Could you check a few things on this model? Use its own coordinates, in mm. A direction names the side the tool comes from. Give positions to 0.01 mm unless a question says otherwise; leave off trailing zeros. Order: outer loops, then holes, each group sorted by start corner. A loop starts at its lowest first (then second) coordinate and runs counter-clockwise, first axis right, second up. Notation, with made-up numbers: M 75,26 L 81,26 A11 cw 81,42 Z; hole C 48,36.5 d2. An arc over 180 degrees is marked long. Answer in a Markdown table with one row per item. Add a question column.
```python
from build123d import *

# Parameters (mm, degrees)
SKETCH_1_R      = 10
EXTRUDE_1_DEPTH = 2.5


with BuildPart() as part:
    # 草图1 → 凸台-拉伸1 (new body)
    with BuildSketch(Plane.XY):
        with BuildLine():
            Line((-24, -40), (-24, -50))
            ThreePointArc((-24, -50), (-15.443695821, -59.895238369), (-4.416851525, -52.857142857))
            ThreePointArc((-4.416851525, -52.857142857), (-2.974049354, -50.792865097), (-0.583592135, -50))
            Line((-0.583592135, -50), (0.583592135, -50))
            ThreePointArc((0.583592135, -50), (2.974049354, -50.792865097), (4.416851525, -52.857142857))
            ThreePointArc((4.416851525, -52.857142857), (15.443695821, -59.895238369), (24, -50))
            Line((24, -50), (24, -40))
            ThreePointArc((24, -40), (23.055385138, -35.757359313), (20.4, -32.316250915))
            ThreePointArc((20.4, -32.316250915), (16.416922293, -27.154588318), (15, -20.790627288))
            Line((15, -20.790627288), (15, 0))
            ThreePointArc((15, 0), (0, 15), (-15, 0))
            Line((-15, 0), (-15, -20.790627288))
            ThreePointArc((-15, -20.790627288), (-16.416922293, -27.154588318), (-20.4, -32.316250915))
            ThreePointArc((-20.4, -32.316250915), (-23.055385138, -35.757359313), (-24, -40))
        make_face()
        Circle(SKETCH_1_R, mode=Mode.SUBTRACT)
        with BuildLine():
            Line((-4.5, -20), (-4.5, -40))
            ThreePointArc((-4.5, -40), (0, -44.5), (4.5, -40))
            Line((4.5, -40), (4.5, -20))
            ThreePointArc((4.5, -20), (0, -15.5), (-4.5, -20))
        make_face(mode=Mode.SUBTRACT)
        with BuildLine():
            ThreePointArc((-17.741657387, -47.5), (-14, -54.5), (-10.258342613, -47.5))
            ThreePointArc((-10.258342613, -47.5), (-9.5, -45), (-10.258342613, -42.5))
            ThreePointArc((-10.258342613, -42.5), (-14, -35.5), (-17.741657387, -42.5))
            ThreePointArc((-17.741657387, -42.5), (-18.5, -45), (-17.741657387, -47.5))
        make_face(mode=Mode.SUBTRACT)
        with BuildLine():
            ThreePointArc((10.258342613, -47.5), (9.5, -45), (10.258342613, -42.5))
            ThreePointArc((10.258342613, -42.5), (14, -35.5), (17.741657387, -42.5))
            ThreePointArc((17.741657387, -42.5), (18.5, -45), (17.741657387, -47.5))
            ThreePointArc((17.741657387, -47.5), (14, -54.5), (10.258342613, -47.5))
        make_face(mode=Mode.SUBTRACT)
    extrude(amount=EXTRUDE_1_DEPTH)


solid = part.part
```
1. Suppose I cut it at A-A on z = 1.4. List the corners of the cut face in (x, y) for me, plus the area to 3 significant figures.
2. Will these pins go through, and if not, where does the flat tip stop? P1, Ø1.5, axis at x = 6.5, z = 2, coming from the -Y side; P2, Ø0.9, axis at x = 0.5, z = 0.5, coming from the -Y side; P3, Ø1.2, axis at y = -28.5, z = 1, coming from the +X side.
3. Suppose I cut it at C-C on y = -22. List the corners of the cut face in (x, z) for me.
4. Thinking about a two-plate mould opening in X: for faces 4 (the cylindrical face through (0, 15, 1)), 5 (the flat face through (4.5, -30, 1)), 6 (the flat face through (24, -45, 1)), which applies, pulls with the +X half, pulls with the -X half, needs draft (parallel to the pull), parting line crosses it, or undercut?
5. Suppose I cut it at B-B on x = -14. List the corners of the cut face in (y, z) for me, plus the area to 3 significant figures.
6. For faces 1 (the flat face through (-6, -30, 0)), 2 (the cylindrical face through (-3, -50.81, 1.23)), 3 (the flat face through (-4.5, -30, 1)), which set-ups out of +Z, -Z, +X, -X, +Y, -Y let a thin tool reach every point of the face, with its end or its side?
7. Suppose I cut it at D-D on x = -3. List the corners of the cut face in (y, z) for me, plus the area to 3 significant figures.
8. If I drill on line 1 along X through (y, z) = (-40, 1.35); line 2 along Y through (x, z) = (-1, 0.8); line 3 along Y through (x, z) = (-13, 2.2), over which ranges is the centre line in solid material (lowest first)? Write a range as [from, to].
Findings below:
| question | item | result |
|---|---|---|
| 1 | outline | M -24,-50 A10 ccw -4.42,-52.86 A4 cw -0.58,-50 L 0.58,-50 A4 cw 4.42,-52.86 A10 ccw 24,-50 L 24,-40 A10 ccw 20.4,-32.32 A15 cw 15,-20.79 L 15,0 A15 ccw -15,0 L -15,-20.79 A15 cw -20.4,-32.32 A10 ccw -24,-40 Z; hole M -17.74,-47.5 A4.5 ccw long -10.26,-47.5 A4.5 ccw -10.26,-42.5 A4.5 ccw long -17.74,-42.5 A4.5 ccw Z; hole C 0,0 d20; hole M -4.5,-40 A4.5 ccw 4.5,-40 L 4.5,-20 A4.5 ccw -4.5,-20 Z; hole M 10.26,-47.5 A4.5 ccw long 17.74,-47.5 A4.5 ccw 17.74,-42.5 A4.5 ccw long 10.26,-42.5 A4.5 ccw Z |
| 1 | area | 1,660 mm2 |
| 2 | P1 | y = -57.38 |
| 2 | P2 | y = -50.02 |
| 2 | P3 | x = 17.51 |
| 3 | outline | M -15.05,0 L -4.5,0 L -4.5,2.5 L -15.05,2.5 Z; M 4.5,0 L 15.05,0 L 15.05,2.5 L 4.5,2.5 Z |
| 4 | face 4 | parting line crosses it |
| 4 | face 5 | undercut |
| 4 | face 6 | pulls with the +X half |
| 5 | outline | M -60,0 L -54.5,0 L -54.5,2.5 L -60,2.5 Z; M -35.5,0 L 5.39,0 L 5.39,2.5 L -35.5,2.5 Z |
| 5 | area | 116 mm2 |
| 6 | face 1 | -Z, +X, -X, +Y, -Y |
| 6 | face 2 | +Z, -Z, -Y |
| 6 | face 3 | +Z, -Z |
| 7 | outline | M -50.81,0 L -43.35,0 L -43.35,2.5 L -50.81,2.5 Z; M -16.65,0 L -9.54,0 L -9.54,2.5 L -16.65,2.5 Z; M 9.54,0 L 14.7,0 L 14.7,2.5 L 9.54,2.5 Z |
| 7 | area | 49.3 mm2 |
| 8 | line 1 | [-24, -18.5], [-9.5, -4.5], [4.5, 9.5], [18.5, 24] |
| 8 | line 2 | [-50.02, -44.39], [-15.61, -9.95], [9.95, 14.97] |
| 8 | line 3 | [-59.95, -54.39], [-35.61, 7.48] |
